Verification items for the finished model (mm, model axes). Face numbers are marked on the shaded views. A direction names the side the tool comes from. Coordinates: 2 decimals unless noted, no trailing zeros. Loops run counter-clockwise (first coordinate to the right, second up) from the corner with the lowest first, then second, coordinate; pieces in that order, holes last. Notation, with made-up numbers: (53.5, -3.5) -> (76.5, -3.5) arc R7 cw to (76.5, 6.5) -> close; hole circle Ø6 at (1.25, 21.25). An arc over 180 degrees is marked (long way). Answer as a JSON object with one key per item and string values. Group by question number.
Q1. Set-up check for the marked faces 4, 5 and 6: record each of +Z, -Z, +X, -X, +Y, -Y from which the full face is reachable in a straight line by a thin tool's end or side.
Q2. Gauge pin test, flat ends, axial feed: pin 1 Ø12 at (x, y) = (-4, 56) entering from -Z; pin 2 Ø12 at (x, z) = (60, 7) entering from -Y; pin 3 Ø10 at (x, z) = (35.5, -3.5) entering from -Y. Record the tip position at first contact, or that the pin passes through.
Q3. Release check for a two-part mould opening along Y. For the marked faces 1, 2 and 3 record: released by +Y, released by -Y, zero draft, split by the parting line, or undercut.
Q4. Scan lines: L1, parallel to Y at x = 0, z = 44.5; L2, parallel to Z at x = -69, y = -38; L3, parallel to Z at x = -50.5, y = -16. Record each from-to range of solid material in increasing order.
Q5. Cross-section at C-C on z = 13. Record the boundary of the cut face in (x, y).
Q6. Cross-section at D-D on y = -63.5. Record the boundary of the cut face in (x, z), and give its area (3 significant figures).
Q7. Cross-section at A-A on y = 0. Record the boundary of the cut face in (x, z), and give its area (3 significant figures).
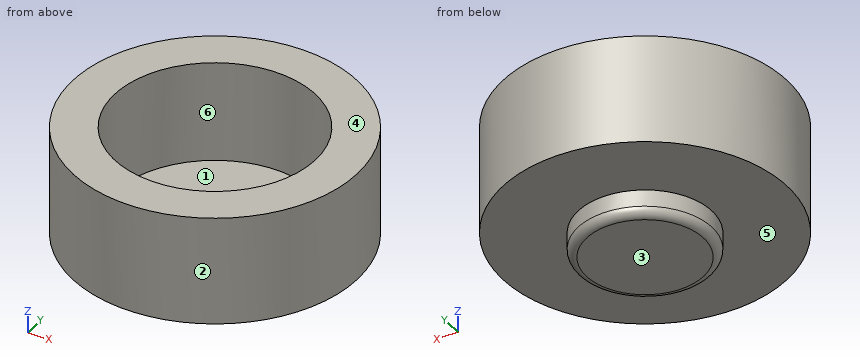
```python
from build123d import *

# Parameters (mm, degrees)
F0_R          = 85
F0_R_2        = 60
F1_DEPTH      = 65
F0_R_3        = 40
F2_DEPTH      = 5
F3_DEPTH      = 5
F3_DEPTH_BACK = 15
F4_R          = 5


with BuildPart() as f1:
    # F0 (on Top) → F1 (new body)
    with BuildSketch(Plane.XY):
        Circle(F0_R)
        Circle(F0_R_2, mode=Mode.SUBTRACT)
    extrude(amount=F1_DEPTH)

    # F0 (on Top) → F2 (join)
    with BuildSketch(Plane.XY):
        Circle(F0_R_2)
        Circle(F0_R_3, mode=Mode.SUBTRACT)
    extrude(amount=F2_DEPTH)

    # F0 (on Top) → F3 (join, two sides)
    with BuildSketch(Plane.XY) as f3_sk:
        Circle(F0_R_3)
    extrude(amount=F3_DEPTH)
    extrude(f3_sk.sketch, amount=-F3_DEPTH_BACK)

    # F4
    f4_edges = [f1.edges().sort_by_distance(p)[0] for p in [
        (-40, 0, -15),
    ]]
    fillet(f4_edges, radius=F4_R)


solid = f1.part
```
Computed values:
{
 "1": {"face 4": "+Z, +X, -X, +Y, -Y", "face 5": "-Z", "face 6": "+Z"},
 "2": {"pin 1": "stops at z = 0", "pin 2": "stops at y = -65.64", "pin 3": "stops at y = -78.78"},
 "3": {"face 1": "undercut", "face 2": "split by the parting line", "face 3": "zero draft"},
 "4": {"L1": "y = -85 to -60, 60 to 85", "L2": "z = 0 to 65", "L3": "z = 0 to 5"},
 "5": {"outline": "circle Ø170 at (0, 0); hole circle Ø120 at (0, 0)"},
 "6": {"outline": "(-56.5, 0) -> (56.5, 0) -> (56.5, 65) -> (-56.5, 65) -> close", "area": "7,350 mm²"},
 "7": {"outline": "(-85, 0) -> (-40, 0) -> (-40, -10) arc R5 ccw to (-35, -15) -> (35, -15) arc R5 ccw to (40, -10) -> (40, 0) -> (85, 0) -> (85, 65) -> (60, 65) -> (60, 5) -> (-60, 5) -> (-60, 65) -> (-85, 65) -> close", "area": "5,040 mm²"}
}
